Geometry check sheet. Reference: drawing and pictorial views, mm from the part's lowest x, y, z. A direction names the side the tool comes from. Give positions to 0.01 mm unless a question says otherwise; leave off trailing zeros. Write each loop counter-clockwise with the first axis right and the second up, starting at its lowest first coordinate (ties: lowest second). Pieces come first, ordered by that corner, then holes. Notation, with made-up numbers: (25, -26.75) -> (76, -26.75) arc R28 cw to (76, -8.75) -> close; hole circle Ø4 at (37.5, 37). An arc over 180 degrees is marked (long way). Return JSON: item names as keys, results as strings.
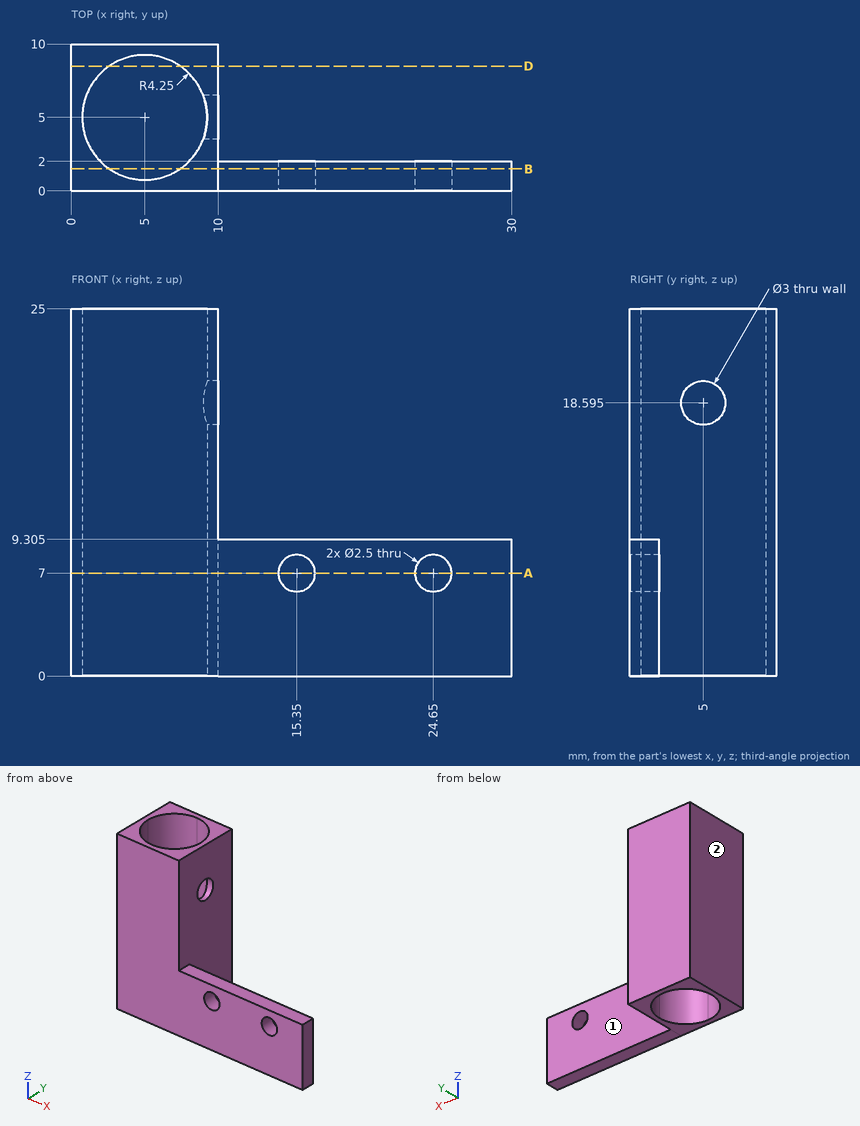
(1) Depth check by flat-ended pin: pin 1 Ø3 at (y, z) = (5, 17) entering from +X; pin 2 Ø6 at (y, z) = (2, 9.5) entering from -X; pin 3 Ø3 at (x, z) = (24.5, 5) entering from +Y; pin 4 Ø2 at (x, y) = (23.5, 1) entering from +Z (1 decimal). Enter the tip coordinate at first touch or a pass-through.
Reply:
{"pin 1": "x = 10", "pin 2": "x = 0", "pin 3": "y = 2", "pin 4": "z = 9.3"}
(2) Cross-section at B-B on y = 1.5. State how many separate pieces and enclosed holes the cut face has, then the cut area to 3 significant figures.
Reply:
{"separate pieces": "2", "enclosed holes": "2", "area": "306 mm^2"}
(3) Cross-section at D-D on y = 8.5. Enter the section's corners in (x, z).
Reply:
{"outline": "(0, 0) -> (2.59, 0) -> (2.59, 25) -> (0, 25) -> close; (7.41, 0) -> (10, 0) -> (10, 25) -> (7.41, 25) -> close"}
(4) Thickness scan on L1, parallel to X at y = 5.25, z = 13.25; L2, parallel to Z at x = 9.5, y = 5 (1 decimal); L3, parallel to Y at x = 5.5, z = 4.5. Record the ranges inside material, lowest first.
Reply:
{"L1": "0 to 0.76, 9.24 to 10", "L2": "0 to 17.1, 20.1 to 25", "L3": "0 to 0.78, 9.22 to 10"}
(5) Set-up check for the marked faces 1 and 2: record each of +Z, -Z, +X, -X, +Y, -Y from which the full face is reachable in a straight line by a thin tool's end or side.
Reply:
{"face 1": "+Z, -Z, +X, +Y", "face 2": "+Z, -Z, -X, +Y, -Y"}
(6) Cross-section at A-A on z = 7. Enter the section's corners in (x, y).
Reply:
{"outline": "(0, 0) -> (14.1, 0) -> (14.1, 2) -> (10, 2) -> (10, 10) -> (0, 10) -> close; (16.6, 0) -> (23.4, 0) -> (23.4, 2) -> (16.6, 2) -> close; (25.9, 0) -> (30, 0) -> (30, 2) -> (25.9, 2) -> close; hole (0.75, 5) arc R4.25 ccw to (5, 0.75) arc R4.25 ccw to (9.25, 5) arc R4.25 ccw to (5, 9.25) arc R4.25 ccw to start"}
